For this review, take the finished solid that the model builds, in its own axes (mm). Give positions to 0.01 mm unless a question says otherwise; leave off trailing zeros. Write item = value, one per line.
```python
from build123d import *

# Parameters (mm, degrees)
BOSS_EXTRUDE1_DEPTH          = 3.175
M4_CLEARANCE_HOLE1_OUTLINE_R = 2.4
M4_CLEARANCE_HOLE1_DEPTH     = 3.175
CUT_EXTRUDE1_DEPTH           = 3.175


# Read off the part's stored shape, not the designer's step: M4 Clearance Hole1
with BuildPart() as part:
    # Sketch2 → Boss-Extrude1 (new body)
    with BuildSketch(Plane.XY):
        with BuildLine():
            Line((227.491320086, -163.756000107), (221.761320086, -163.756000107))
            ThreePointArc((221.761320086, -163.756000107), (219.516256056, -162.826064137), (218.586320086, -160.581000107))
            Line((218.586320086, -160.581000107), (218.586320086, -157.216000107))
            Line((218.586320086, -157.216000107), (149.097320094, -157.216000107))
            Line((149.097320094, -157.216000107), (149.097320094, -160.581000107))
            ThreePointArc((149.097320094, -160.581000107), (148.167384125, -162.826064137), (145.922320094, -163.756000107))
            Line((145.922320094, -163.756000107), (140.192320094, -163.756000107))
            ThreePointArc((140.192320094, -163.756000107), (137.947256064, -162.826064137), (137.017320094, -160.581000107))
            Line((137.017320094, -160.581000107), (137.017320094, -157.216000107))
            Line((137.017320094, -157.216000107), (49.052320094, -157.216000107))
            Line((49.052320094, -157.216000107), (49.052320094, -160.581000107))
            ThreePointArc((49.052320094, -160.581000107), (48.122384125, -162.826064137), (45.877320094, -163.756000107))
            Line((45.877320094, -163.756000107), (40.147320094, -163.756000107))
            ThreePointArc((40.147320094, -163.756000107), (37.902256064, -162.826064137), (36.972320094, -160.581000107))
            Line((36.972320094, -160.581000107), (36.972320094, -157.216000107))
            Line((36.972320094, -157.216000107), (-32.516679898, -157.216000107))
            Line((-32.516679898, -157.216000107), (-32.516679898, -160.581000107))
            ThreePointArc((-32.516679898, -160.581000107), (-33.446615867, -162.826064137), (-35.691679898, -163.756000107))
            Line((-35.691679898, -163.756000107), (-41.421679898, -163.756000107))
            ThreePointArc((-41.421679898, -163.756000107), (-43.666743928, -162.826064137), (-44.596679898, -160.581000107))
            Line((-44.596679898, -160.581000107), (-44.596679898, -157.216000107))
            Line((-44.596679898, -157.216000107), (-132.561679898, -157.216000107))
            Line((-132.561679898, -157.216000107), (-132.561679898, -160.581000107))
            ThreePointArc((-132.561679898, -160.581000107), (-133.491615867, -162.826064137), (-135.736679898, -163.756000107))
            Line((-135.736679898, -163.756000107), (-141.466679898, -163.756000107))
            ThreePointArc((-141.466679898, -163.756000107), (-143.711743928, -162.826064137), (-144.641679898, -160.581000107))
            Line((-144.641679898, -160.581000107), (-144.641679898, -157.216000107))
            Line((-144.641679898, -157.216000107), (-174.499179878, -157.216000107))
            Line((-174.499179878, -157.216000107), (-174.499179878, -167.122000107))
            Line((-174.499179878, -167.122000107), (-172.356179878, -167.122000107))
            Line((-172.356179878, -167.122000107), (-172.356179878, -168.265000107))
            Line((-172.356179878, -168.265000107), (-173.499179878, -168.265000107))
            Line((-173.499179878, -168.265000107), (-173.499179878, -193.665000107))
            Line((-173.499179878, -193.665000107), (-172.356179878, -193.665000107))
            Line((-172.356179878, -193.665000107), (-172.356179878, -194.181000107))
            Line((-172.356179878, -194.181000107), (-154.179179878, -194.181000107))
            Line((-154.179179878, -194.181000107), (-154.179179878, -203.714000107))
            Line((-154.179179878, -203.714000107), (249.446820082, -203.714000107))
            Line((249.446820082, -203.714000107), (249.446820082, -194.181000107))
            Line((249.446820082, -194.181000107), (267.623820082, -194.181000107))
            Line((267.623820082, -194.181000107), (267.623820082, -193.665000107))
            Line((267.623820082, -193.665000107), (268.766820082, -193.665000107))
            Line((268.766820082, -193.665000107), (268.766820082, -168.265000107))
            Line((268.766820082, -168.265000107), (267.623820082, -168.265000107))
            Line((267.623820082, -168.265000107), (267.623820082, -167.122000107))
            Line((267.623820082, -167.122000107), (269.766820082, -167.122000107))
            Line((269.766820082, -167.122000107), (269.766820082, -157.216000107))
            Line((269.766820082, -157.216000107), (230.666320086, -157.216000107))
            Line((230.666320086, -157.216000107), (230.666320086, -160.581000107))
            ThreePointArc((230.666320086, -160.581000107), (229.736384117, -162.826064137), (227.491320086, -163.756000107))
        make_face()
    extrude(amount=BOSS_EXTRUDE1_DEPTH)

    # M4 Clearance Hole1 outline → M4 Clearance Hole1 (cut)
    with BuildSketch(Plane.XY):
        with Locations((233.170320102, -183.106000107)):
            Circle(M4_CLEARANCE_HOLE1_OUTLINE_R)
        with Locations((186.970320102, -183.106000107)):
            Circle(M4_CLEARANCE_HOLE1_OUTLINE_R)
        with Locations((114.745320102, -165.106000107)):
            Circle(M4_CLEARANCE_HOLE1_OUTLINE_R)
        with Locations((65.745320102, -165.106000107)):
            Circle(M4_CLEARANCE_HOLE1_OUTLINE_R)
        with Locations((-97.702679898, -181.106000107)):
            Circle(M4_CLEARANCE_HOLE1_OUTLINE_R)
        with Locations((-143.902679898, -181.106000107)):
            Circle(M4_CLEARANCE_HOLE1_OUTLINE_R)
    extrude(amount=M4_CLEARANCE_HOLE1_DEPTH, mode=Mode.SUBTRACT)

    # Sketch5 → Cut-Extrude1 (cut)
    with BuildSketch(Plane.XY.offset(3.175)):
        Polygon((264.766820082, -175.717058259), (268.766820082, -175.717058259), (268.766820082, -176.460000107), (266.515167585, -176.460000107), (264.766820082, -176.928468408), align=None)
        with BuildLine():
            Line((271.531820082, -185.652747691), (271.531820082, -186.212941955))
            Line((271.531820082, -186.212941955), (268.766820082, -186.212941955))
            Line((268.766820082, -186.212941955), (268.766820082, -185.470000107))
            Line((268.766820082, -185.470000107), (266.515167585, -185.470000107))
            Line((266.515167585, -185.470000107), (264.766820082, -185.001531806))
            Line((264.766820082, -185.001531806), (264.766820082, -176.928468408))
            Line((264.766820082, -176.928468408), (266.515167585, -176.460000107))
            Line((266.515167585, -176.460000107), (268.766820082, -176.460000107))
            Line((268.766820082, -176.460000107), (268.766820082, -175.717058259))
            Line((268.766820082, -175.717058259), (271.531820082, -175.717058259))
            Line((271.531820082, -175.717058259), (271.531820082, -176.277252523))
            ThreePointArc((271.531820082, -176.277252523), (272.085217516, -176.676347658), (272.296820082, -177.325000107))
            Line((272.296820082, -177.325000107), (272.296820082, -184.605000107))
            ThreePointArc((272.296820082, -184.605000107), (272.085217516, -185.253652556), (271.531820082, -185.652747691))
        make_face()
        Polygon((264.766820082, -185.001531806), (264.766820082, -186.212941955), (268.766820082, -186.212941955), (268.766820082, -185.470000107), (266.515167585, -185.470000107), align=None)
    cut_extrude1 = extrude(amount=-CUT_EXTRUDE1_DEPTH, mode=Mode.SUBTRACT)

    # Mirror1: Cut-Extrude1 across plane
    add(cut_extrude1.mirror(Plane(origin=(47.633820102, 0, 0), x_dir=(0, 0, 1), z_dir=(1, 0, 0))), mode=Mode.SUBTRACT)


solid = part.part
```
(1) Take a section at A-A (z = 1.1). Count the separate pieces of the cut face and the enclosed holes in it, plus the area to 3 significant figures.
Answers below:
separate_pieces = 1
enclosed_holes = 6
area = 19,600 mm^2
(2) To check wall thickness, follow probe 1 along X at (y, z) = (-180.5, 2.2); probe 2 along X at (y, z) = (-185, 1.6); probe 3 along X at (y, z) = (-168, 0.6). State the ranges of each line that lie inside material, in increasing order.
Answers below:
probe_1 = -169.5 to -146.22, -141.58 to -100.02, -95.38 to 264.77
probe_2 = -169.5 to 185.5, 188.44 to 231.7, 234.64 to 264.77
probe_3 = -172.36 to 267.62
(3) For pin 1 (1.6 mm diameter, centred on y = -188, z = 1, fed in from +X), flat-tipped, find the tip position at first contact; note if it passes through.
Answers below:
pin_1 = 268.77
